from build123d import *

# Parameters (mm, degrees)
F0_W     = 67.591384
F0_H     = 48.631672
F1_DEPTH = 72.644
F3_D     = 25.4
F5_D     = 25.4


with BuildPart() as f1:
    # F0 (on Front) → F1 (new body)
    with BuildSketch(Plane.XZ):
        with Locations((33.795692, 24.315836)):
            Rectangle(F0_W, F0_H)
    extrude(amount=F1_DEPTH)

    # F3 (through all)
    with Locations(Plane.XY.offset(48.631672)):
        with Locations((27.831206, -42.929504)):
            Hole(F3_D / 2)

    # F5 (through all)
    with Locations(Plane(origin=(0, 0, 0), x_dir=(0, -1, 0), z_dir=(-1, 0, 0))):
        with Locations((35.879802, 23.983832)):
            Hole(F5_D / 2)


solid = f1.part
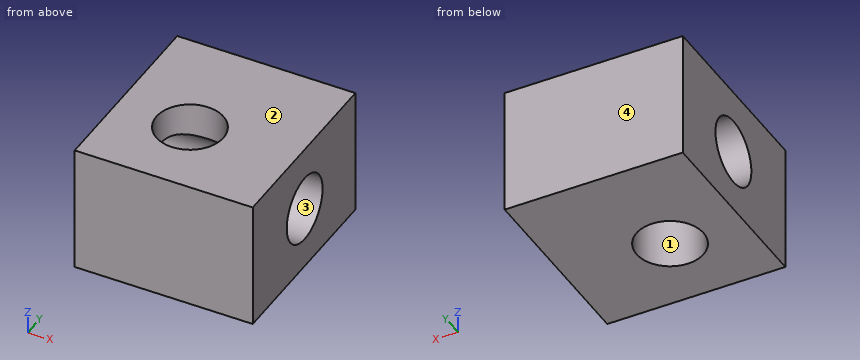
For this review, take the finished solid that the model builds, in its own axes (mm). Face numbers are marked on the shaded views. Coordinates: 2 decimals unless noted, no trailing zeros. Order: outer loops, then holes, each group sorted by start corner. A loop starts at its lowest first (then second) coordinate and runs counter-clockwise, first axis right, second up. Notation, with made-up numbers: (70, 36.25) - (129, 36.25) arc R36 cw to (129, 71.25) - close; hole circle Ø8 at (30.25, 16.25). An arc over 180 degrees is marked (long way). Use one line per item in the form item = value.
Q1. Consider section C-C (y = -37.5). Give the boundary of the cut face in (x, z), then the cut area to 3 significant figures.
Checked values:
outline = (0, 0) - (16.35, 0) - (16.35, 11.39) - (0, 11.39) - close; (0, 36.58) - (16.35, 36.58) - (16.35, 48.63) - (0, 48.63) - close; (39.31, 0) - (67.59, 0) - (67.59, 11.39) - (39.31, 11.39) - close; (39.31, 36.58) - (67.59, 36.58) - (67.59, 48.63) - (39.31, 48.63) - close
area = 1,050 mm2
Q2. Consider section A-A (y = -28). Give the boundary of the cut face in (x, z), then the cut area to 3 significant figures.
Checked values:
outline = (0, 0) - (67.59, 0) - (67.59, 14.02) - (0, 14.02) - close; (0, 33.94) - (67.59, 33.94) - (67.59, 48.63) - (0, 48.63) - close
area = 1,940 mm2
Q3. Consider section D-D (z = 8). Give the boundary of the cut face in (x, y).
Checked values:
outline = (0, -72.64) - (67.59, -72.64) - (67.59, 0) - (0, 0) - close; hole circle Ø25.4 at (27.83, -42.93)
Q4. Draft analysis for pull direction Y (two halves, no side actions). For the marked faces 1, 2, 3 and 4, state which applies: +Y half, -Y half, draft (parallel to the pull), parting line (faces both ways), or undercut.
Checked values:
face_1 = undercut
face_2 = draft
face_3 = undercut
face_4 = +Y half
Q5. Consider section B-B (x = 17). Give the boundary of the cut face in (y, z), then the cut area to 3 significant figures.
Checked values:
outline = (-72.64, 0) - (-49.56, 0) - (-49.56, 48.63) - (-72.64, 48.63) - close; (-36.3, 0) - (0, 0) - (0, 48.63) - (-36.3, 48.63) - (-36.3, 36.68) arc R12.7 cw (long way) to (-36.3, 11.29) - close
area = 2,620 mm2
Q6. For probe 1 along X at (y, z) = (-42.5, 40.5); probe 2 along Y at (x, z) = (9, 12.5); probe 3 along X at (y, z) = (-39.5, 40), list the stretches that pass through material, from the lowest coordinate up. Write a range as from..to.
Checked values:
probe_1 = 0..15.14, 40.52..67.59
probe_2 = -72.64..-41.3, -30.46..0
probe_3 = 0..15.6, 40.06..67.59
